```python
from build123d import *

# Parameters (mm, degrees)
SKETCH1_W           = 30
SKETCH1_H           = 30
BOSS_EXTRUDE1_DEPTH = 30
SHELL1_T            = -2
SKETCH2_R           = 6
CUT_EXTRUDE1_DEPTH  = 40
SKETCH3_R           = 6
CUT_EXTRUDE2_DEPTH  = 40


with BuildPart() as part:
    # Sketch1 → Boss-Extrude1 (new body)
    with BuildSketch(Plane(origin=(0, 0, 0), x_dir=(0, 1, 0), z_dir=(0, 0, 1))):
        Rectangle(SKETCH1_W, SKETCH1_H)
    extrude(amount=BOSS_EXTRUDE1_DEPTH)

    # Shell1
    shell1_openings = [part.faces().sort_by_distance(p)[0] for p in [
        (0, 0, 30),
    ]]
    offset(amount=SHELL1_T, openings=shell1_openings, kind=Kind.INTERSECTION)

    # Sketch2 → Cut-Extrude1 (cut)
    with BuildSketch(Plane(origin=(0, 15, 0), x_dir=(-1, 0, 0), z_dir=(0, 1, 0))):
        with Locations((0, 15)):
            Circle(SKETCH2_R)
    extrude(amount=-CUT_EXTRUDE1_DEPTH, mode=Mode.SUBTRACT)

    # Sketch3 → Cut-Extrude2 (cut)
    with BuildSketch(Plane.YZ.offset(15)):
        with Locations((0, 15)):
            Circle(SKETCH3_R)
    extrude(amount=-CUT_EXTRUDE2_DEPTH, mode=Mode.SUBTRACT)


solid = part.part
```
The listing builds one solid part. Answer for the finished solid, in the listing's coordinates (mm). A direction names the side the tool comes from. Coordinates: 2 decimals unless noted, no trailing zeros. Write each loop counter-clockwise with the first axis right and the second up, starting at its lowest first coordinate (ties: lowest second). Pieces come first, ordered by that corner, then holes. Notation, with made-up numbers: (46, 88.5) - (96, 88.5) arc R21 ccw to (96, 95.5) - close; hole circle Ø11 at (44, -35). An arc over 180 degrees is marked (long way). One line per item, written item: value.
1) For a pull along Y with two mould halves and no side action, classify faces 1 (the flat face through (0, 13, 22)), 2 (the flat face through (0, 15, 8)), 3 (the flat face through (-13, 0, 22)), 4 (the flat face through (-15, 0, 8)) as pulls with the +Y half, pulls with the -Y half, needs draft (parallel to the pull), parting line crosses it, or undercut.
Geometry check:
face 1: undercut
face 2: pulls with the +Y half
face 3: undercut
face 4: needs draft
2) A tool of negligible diameter and unlimited length cuts with its end or side. For faces 5 (the cylindrical face through (6, 14, 15)), 6 (the flat face through (13, 0, 22)), from which of +Z, -Z, +X, -X, +Y, -Y can it reach the whole face along a straight path? Write none if from no direction.
Geometry check:
face 5: +Y, -Y
face 6: +Z
3) Each of these flat-tipped pins is pushed along its axis until it touches: pin 1 Ø1 at (y, z) = (4.5, 14) entering from +X; pin 2 Ø8 at (x, y) = (3.5, -0.5) entering from +Z. Where does it stop, or does it pass through?
Geometry check:
pin 1: passes through
pin 2: stops at z = 2
4) Find section B-B (z = 2.5). Give the vertices of the cut face in (x, y), and give its area (3 significant figures).
Geometry check:
outline: (-15, -15) - (15, -15) - (15, 15) - (-15, 15) - close; hole (-13, -13) - (13, -13) - (13, 13) - (-13, 13) - close
area: 224 mm2
5) Find section D-D (z = 15). Give the vertices of the cut face in (x, y).
Geometry check:
outline: (-15, -15) - (-6, -15) - (-6, -13) - (-13, -13) - (-13, -6) - (-15, -6) - close; (-15, 6) - (-13, 6) - (-13, 13) - (-6, 13) - (-6, 15) - (-15, 15) - close; (6, -15) - (15, -15) - (15, -6) - (13, -6) - (13, -13) - (6, -13) - close; (6, 13) - (13, 13) - (13, 6) - (15, 6) - (15, 15) - (6, 15) - close
6) Find section A-A (y = 0). Give the vertices of the cut face in (x, z), and give its area (3 significant figures).
Geometry check:
outline: (-15, 0) - (15, 0) - (15, 9) - (13, 9) - (13, 2) - (-13, 2) - (-13, 9) - (-15, 9) - close; (-15, 21) - (-13, 21) - (-13, 30) - (-15, 30) - close; (13, 21) - (15, 21) - (15, 30) - (13, 30) - close
area: 124 mm2
7) Consider line 1 along Z through (x, y) = (0, -13.9); line 2 along X through (y, z) = (-3, 21.25). Determine where each line is inside the solid, lowest interval first. Write a range as from..to.
Geometry check:
line 1: z = 0..9, 21..30
line 2: x = -15..-13, 13..15
